Check sheet for the modelled part. Datum: model origin and axes. Units: mm. Face numbers are marked on the shaded views. A direction names the side the tool comes from. Give positions to 0.01 mm unless a question says otherwise; leave off trailing zeros. Loops run counter-clockwise (first coordinate to the right, second up) from the corner with the lowest first, then second, coordinate; pieces in that order, holes last. Notation, with made-up numbers: (29.25, 49) -> (34.25, 49) arc R8 ccw to (34.25, 56) -> close; hole circle Ø4 at (12, -37). An arc over 180 degrees is marked (long way). Write each question's results on one line, items separated by ' | '. Start each with the question number.
Item 1: Scan lines: line 1 along Z through (x, y) = (36, 2.5); line 2 along X through (y, z) = (-10, 8); line 3 along X through (y, z) = (-8.5, 3.5). Record each from-to range of solid material in increasing order.
Item 2: Cross-section at B-B on x = 27.5. Enter the section's corners in (y, z), then the cut area to 3 significant figures.
Item 3: Cross-section at A-A on z = 0. Enter the section's corners in (x, y).
Item 4: Gauge pin test, flat ends, axial feed: pin 1 Ø6 at (x, z) = (7.5, -3) entering from -Y; pin 2 Ø3 at (y, z) = (4.5, 3.5) entering from +X; pin 3 Ø5 at (x, z) = (38.5, -7) entering from -Y. Record the tip position at first contact, or that the pin passes through.
Item 5: Cross-section at D-D on x = 22. Enter the section's corners in (y, z), then the cut area to 3 significant figures.
Item 6: Mould release check, pull along Z, two halves, no side actions. Record for the marked faces 4, 5, 6 and 7: pulls with the +Z half, pulls with the -Z half, needs draft (parallel to the pull), parting line crosses it, or undercut.
Item 7: Access from +Z, -Z, +X, -X, +Y, -Y to the whole of each face (thin tool, end or side, straight path). Record for the marked faces 1, 2 and 3.
Item 8: Cross-section at C-C on y = 0. Enter the section's corners in (x, z).
from build123d import *

# Parameters (mm, degrees)
SKETCH_1_R          = 10
EXTRUDE_1_DEPTH     = 3.5
SKETCH_2_W          = 24
SKETCH_2_H          = 30
EXTRUDE_2_DEPTH     = 2
SKETCH_3_W          = 2
SKETCH_3_H          = 30
EXTRUDE_3_DEPTH     = 40
CUT_EXTRUDE_1_DEPTH = 40
FILLET_1_R          = 2
SKETCH_5_R          = 1.5
EXTRUDE_4_DEPTH     = 24


with BuildPart() as part:
    # 草图1 → 凸台-拉伸1 (new body)
    with BuildSketch(Plane(origin=(0, 0, 0), x_dir=(0, 0, -1), z_dir=(1, 0, 0))):
        Circle(SKETCH_1_R)
    extrude(amount=EXTRUDE_1_DEPTH)

    # 草图2 → 凸台-拉伸2 (add)
    with BuildSketch(Plane(origin=(3.5, 0, 0), x_dir=(0, 0, -1), z_dir=(1, 0, 0))):
        Rectangle(SKETCH_2_W, SKETCH_2_H)
    extrude(amount=EXTRUDE_2_DEPTH)

    # 草图3 → 凸台-拉伸3 (add)
    with BuildSketch(Plane(origin=(5.5, 0, 0), x_dir=(0, 0, -1), z_dir=(1, 0, 0))):
        with Locations((11, 0)):
            Rectangle(SKETCH_3_W, SKETCH_3_H)
        with Locations((-11, 0)):
            Rectangle(SKETCH_3_W, SKETCH_3_H)
    extrude(amount=EXTRUDE_3_DEPTH)

    # 草图4 → 切除-拉伸1 (cut)
    with BuildSketch(Plane.XY.offset(12)):
        with BuildLine():
            Line((45.5, 5.517073487), (45.5, 15))
            Line((45.5, 15), (3.5, 15))
            ThreePointArc((3.5, 15), (24.928800083, 12.157697667), (45.5, 5.517073487))
        make_face()
        with BuildLine():
            Line((3.5, -15), (45.5, -15))
            Line((45.5, -15), (45.5, -5.517073487))
            ThreePointArc((45.5, -5.517073487), (24.928800083, -12.157697667), (3.5, -15))
        make_face()
    extrude(amount=-CUT_EXTRUDE_1_DEPTH, mode=Mode.SUBTRACT)

    # 圆角1
    fillet_1_edges = [part.edges().sort_by_distance(p)[0] for p in [
        (45.5, -5.517073487, 11),
        (45.5, 5.517073487, 11),
        (45.5, 5.517073487, -11),
        (45.5, -5.517073487, -11),
    ]]
    fillet(fillet_1_edges, radius=FILLET_1_R)

    # 草图5 → 凸台-拉伸4 (add)
    with BuildSketch(Plane.XY.offset(12)):
        with Locations(Location((33.5, 0, 0), (0, 0, 270))):
            Circle(SKETCH_5_R)
    extrude(amount=-EXTRUDE_4_DEPTH)


solid = part.part
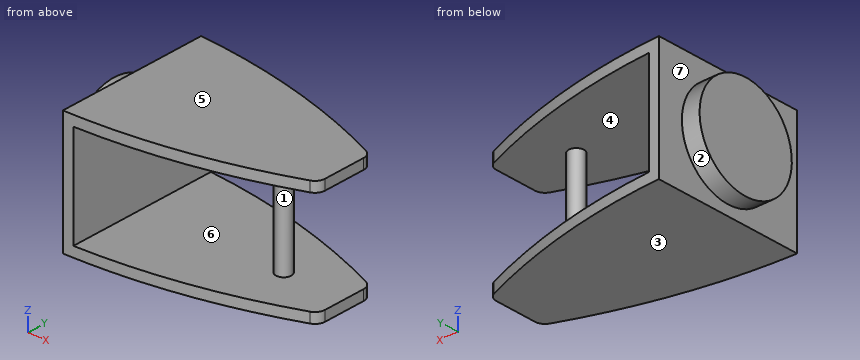
Answer sheet:
1) line 1: z = -12 to -10, 10 to 12 | line 2: x = 3.5 to 5.5 | line 3: x = 0 to 5.5
2) outline: (-11.55, -12) -> (11.55, -12) -> (11.55, -10) -> (-11.55, -10) -> close; (-11.55, 10) -> (11.55, 10) -> (11.55, 12) -> (-11.55, 12) -> close | area: 92.4 mm²
3) outline: (0, -10) -> (3.5, -10) -> (3.5, -15) arc R120 ccw to (5.5, -14.9) -> (5.5, 14.9) arc R120 ccw to (3.5, 15) -> (3.5, 10) -> (0, 10) -> close; circle Ø3 at (33.5, 0)
4) pin 1: stops at y = -14.95 | pin 2: stops at x = 5.5 | pin 3: passes through
5) outline: (-12.78, -12) -> (12.78, -12) -> (12.78, -10) -> (-12.78, -10) -> close; (-12.78, 10) -> (12.78, 10) -> (12.78, 12) -> (-12.78, 12) -> close | area: 102 mm²
6) face 4: undercut | face 5: pulls with the +Z half | face 6: undercut | face 7: needs draft
7) face 1: none | face 2: -X | face 3: -Z, +X, -X, +Y, -Y
8) outline: (0, -10) -> (3.5, -10) -> (3.5, -12) -> (45.5, -12) -> (45.5, -10) -> (35, -10) -> (35, 10) -> (45.5, 10) -> (45.5, 12) -> (3.5, 12) -> (3.5, 10) -> (0, 10) -> close; hole (5.5, -10) -> (32, -10) -> (32, 10) -> (5.5, 10) -> close
